```python
from build123d import *

# Parameters (mm, degrees)
CROQUIS1_W              = 60
CROQUIS1_H              = 60
SALIENTE_EXTRUIR1_DEPTH = 3
REDONDEO1_R             = 2
CROQUIS2_W              = 24
CROQUIS2_H              = 24
SALIENTE_EXTRUIR2_DEPTH = 5
SALIENTE_EXTRUIR2_TAPER = 60
SALIENTE_EXTRUIR3_DEPTH = 3.5
CROQUIS7_R              = 2
CORTAR_EXTRUIR1_DEPTH   = 7


with BuildPart() as part:
    # Croquis1 → Saliente-Extruir1 (new body)
    with BuildSketch(Plane.XY):
        Rectangle(CROQUIS1_W, CROQUIS1_H)
    extrude(amount=SALIENTE_EXTRUIR1_DEPTH)

    # Redondeo1
    redondeo1_edges = [part.edges().sort_by_distance(p)[0] for p in [
        (-30, 0, 3),
        (0, -30, 3),
        (30, 0, 3),
        (0, 30, 3),
    ]]
    fillet(redondeo1_edges, radius=REDONDEO1_R)

    # Croquis2 → Saliente-Extruir2 (add)
    with BuildSketch(Plane.XY.offset(3)):
        Rectangle(CROQUIS2_W, CROQUIS2_H)
    extrude(amount=SALIENTE_EXTRUIR2_DEPTH, taper=SALIENTE_EXTRUIR2_TAPER)

    # Croquis6 → Saliente-Extruir3 (add, symmetric)
    with BuildSketch(Plane(origin=(0, 0, 0), x_dir=(1, 0, 0), z_dir=(0, 1, 0))):
        with BuildLine():
            Line((-3.339745962, -8), (-3.339745962, -13.130693005))
            ThreePointArc((-3.339745962, -13.130693005), (0, -16.470438967), (3.339745962, -13.130693005))
            Line((3.339745962, -13.130693005), (3.339745962, -8))
            Line((3.339745962, -8), (-3.339745962, -8))
        make_face()
    extrude(amount=SALIENTE_EXTRUIR3_DEPTH, both=True)

    # Croquis7 → Cortar-Extruir1 (cut)
    with BuildSketch(Plane.XZ.offset(3.5)):
        with Locations(Location((0, 13.130693005, 0), (0, 0, 270))):
            Circle(CROQUIS7_R)
    extrude(amount=-CORTAR_EXTRUIR1_DEPTH, mode=Mode.SUBTRACT)


solid = part.part
```
Source: CAD feature listing. Evaluate the final solid. Frame: model axes, mm. A direction names the side the tool comes from. Give positions to 0.01 mm unless a question says otherwise; leave off trailing zeros. Loops run counter-clockwise (first coordinate to the right, second up) from the corner with the lowest first, then second, coordinate; pieces in that order, holes last. Notation, with made-up numbers: M -16,-17.5 L 36,-17.5 A12 cw 36,-11.5 Z; hole C 35.25,64.25 d10. An arc over 180 degrees is marked long. Put each result on its own line as item: value.
Q1. Section A-A (x = 0). Return the cut outline in (y, z), and give its area (3 significant figures).
Response values:
outline: M -30,0 L 30,0 L 30,1 A2 ccw 28,3 L 12,3 L 3.34,8 L 3.5,8 L 3.5,11.13 L -3.5,11.13 L -3.5,8 L -3.34,8 L -12,3 L -28,3 A2 ccw -30,1 Z; M -3.5,15.13 L 3.5,15.13 L 3.5,16.47 L -3.5,16.47 Z
area: 286 mm²
Q2. Line query: probe 1 along Z at (x, y) = (10, -25.5); probe 2 along X at (y, z) = (25.5, 1.25); probe 3 along X at (y, z) = (-3, 12.5). Output: solid intervals per line, ascending. Write a range as [from, to].
Response values:
probe 1: z = [0, 3]
probe 2: x = [-29.98, 29.98]
probe 3: x = [-3.34, -1.9], [1.9, 3.34]
Q3. Section C-C (x = 6). Return the cut outline in (y, z).
Response values:
outline: M -30,0 L 30,0 L 30,1 A2 ccw 28,3 L 12,3 L 6,6.46 L -6,6.46 L -12,3 L -28,3 A2 ccw -30,1 Z
Q4. Section B-B (y = 0.5). Return the cut outline in (x, z).
Response values:
outline: M -30,0 L 30,0 L 30,1 A2 ccw 28,3 L 12,3 L 3.34,8 L 3.34,13.13 A3.34 ccw -3.34,13.13 L -3.34,8 L -12,3 L -28,3 A2 ccw -30,1 Z; hole C 0,13.13 d4
Q5. Mould query, pull axis Z, two halves, no side actions, for faces 1 (the cylindrical face through (-1.952, -0.049, 13.564)), 2 (the flat face through (-1, 3.5, 11)), 3 (the flat face through (0, 0, 0)). Classes: released by +Z, released by -Z, zero draft, split by the parting line, or undercut.
Response values:
face 1: undercut
face 2: zero draft
face 3: released by -Z
Q6. Reachability of faces 4 (the flat face through (-1, -3.5, 11)), 5 (the flat face through (-3.34, 0, 11)), 6 (the flat face through (3.34, 0, 11)), 7 (the flat face through (-13, 0, 3)), 8 (the cylindrical face through (0.42, 29.43, 2.4)) from +Z, -Z, +X, -X, +Y, -Y: full face, straight path, thin tool, end or side. Return the list, or none.
Response values:
face 4: +Z, +X, -X, -Y
face 5: +Z, -X, +Y, -Y
face 6: +Z, +X, +Y, -Y
face 7: +Z
face 8: +Z, +X, -X, +Y
Q7. Section D-D (z = 8.75). Return the cut outline in (x, y).
Response values:
outline: M -3.34,-3.5 L 3.34,-3.5 L 3.34,3.5 L -3.34,3.5 Z
Q8. Pin query (flat end, axial travel): P1, Ø1.5, axis at x = -9.5, y = -8.5, coming from the +Z side; P2, Ø4, axis at x = -12.5, y = 17.5, coming from the +Z side; P3, Ø3, axis at x = -2, z = 6.5, coming from the +Y side; P4, Ø1.5, axis at x = 17.5, z = 5, coming from the -Y side. Return the tip coordinate at first contact, or that it passes through.
Response values:
P1: stops at z = 4.88
P2: stops at z = 3
P3: stops at y = 8.54
P4: passes through
